Check sheet for the modelled part. Datum: model origin and axes. Units: mm. A direction names the side the tool comes from. Coordinates: 2 decimals unless noted, no trailing zeros. Loops run counter-clockwise (first coordinate to the right, second up) from the corner with the lowest first, then second, coordinate; pieces in that order, holes last. Notation, with made-up numbers: M 7,75 L 30,75 A30 cw 30,100 Z; hole C 80,88 d2. An arc over 180 degrees is marked long. Return JSON: item names as keys, results as strings.
from build123d import *

# Parameters (mm, degrees)
F0_W     = 9.52
F0_H     = 4.8375
F1_DEPTH = 1.5
F2_W     = 1.7
F2_H     = 6.7225
F3_DEPTH = 1.501


with BuildPart() as f1:
    # F0 (on Top) → F1 (new body)
    with BuildSketch(Plane.XY):
        with Locations((0, 8.88625)):
            Rectangle(F0_W, F0_H)
        with BuildLine():
            ThreePointArc((17.96, -4.5625), (13.3975, 0), (17.96, 4.5625))
            Line((17.96, 4.5625), (17.96, 6.4675))
            ThreePointArc((17.96, 6.4675), (11.4925, 0), (17.96, -6.4675))
            Line((17.96, -6.4675), (17.96, -4.5625))
        make_face()
        with BuildLine():
            Line((-17.96, -4.5625), (-17.96, -6.4675))
            ThreePointArc((-17.96, -6.4675), (-13.386787, -4.573213), (-11.4925, 0))
            ThreePointArc((-11.4925, 0), (-13.386787, 4.573213), (-17.96, 6.4675))
            Line((-17.96, 6.4675), (-17.96, 4.5625))
            ThreePointArc((-17.96, 4.5625), (-14.733825, 3.226175), (-13.3975, 0))
            ThreePointArc((-13.3975, 0), (-14.733825, -3.226175), (-17.96, -4.5625))
        make_face()
        with BuildLine():
            ThreePointArc((17.96, 4.5625), (21.186175, 3.226175), (22.5225, 0))
            ThreePointArc((22.5225, 0), (21.186175, -3.226175), (17.96, -4.5625))
            Line((17.96, -4.5625), (17.96, -6.4675))
            ThreePointArc((17.96, -6.4675), (22.533213, -4.573213), (24.4275, 0))
            ThreePointArc((24.4275, 0), (22.533213, 4.573213), (17.96, 6.4675))
            Line((17.96, 6.4675), (17.96, 4.5625))
        make_face()
        with BuildLine():
            ThreePointArc((-17.96, 6.4675), (-24.4275, 0), (-17.96, -6.4675))
            Line((-17.96, -6.4675), (-17.96, -4.5625))
            ThreePointArc((-17.96, -4.5625), (-22.5225, 0), (-17.96, 4.5625))
            Line((-17.96, 4.5625), (-17.96, 6.4675))
        make_face()
        with BuildLine():
            ThreePointArc((17.96, -6.4675), (11.4925, 0), (17.96, 6.4675))
            Line((17.96, 6.4675), (4.76, 6.4675))
            Line((4.76, 6.4675), (-4.76, 6.4675))
            Line((-4.76, 6.4675), (-17.96, 6.4675))
            ThreePointArc((-17.96, 6.4675), (-13.386787, 4.573213), (-11.4925, 0))
            ThreePointArc((-11.4925, 0), (-13.386787, -4.573213), (-17.96, -6.4675))
            Line((-17.96, -6.4675), (17.96, -6.4675))
        make_face()
    extrude(amount=F1_DEPTH)

    # F2 (on face) → F3 (cut, through all)
    with BuildSketch(Plane.XY.offset(1.5)):
        with Locations((0, -3.10625)):
            Rectangle(F2_W, F2_H)
    extrude(amount=-F3_DEPTH, mode=Mode.SUBTRACT)


solid = f1.part
1) Set-up check for faces 1 (the face through (0.85, -3, 1)), 2 (the face through (-24.426, 0.142, 0.74)), 3 (the face through (-11, 6.468, 1)), 4 (the face through (11, 6.468, 1)): record each of +Z, -Z, +X, -X, +Y, -Y from which the full face is reachable in a straight line by a thin tool's end or side.
Answers:
{"face 1": "+Z, -Z, -Y", "face 2": "+Z, -Z, -X", "face 3": "+Z, -Z, -X, +Y", "face 4": "+Z, -Z, +X, +Y"}
2) Section check D-D on x = -9. Record the cut outline in (y, z), then the cut area to 3 significant figures.
Answers:
{"outline": "M -6.47,0 L 6.47,0 L 6.47,1.5 L -6.47,1.5 Z", "area": "19.4 mm²"}
3) Go/stop test with flat-tipped pins: pin 1 Ø10 at (x, y) = (12, 4.5) entering from -Z; pin 2 Ø0.8 at (y, z) = (8, 0.5) entering from +X. Record where each tip stops, or that it passes through.
Answers:
{"pin 1": "z = 0", "pin 2": "x = 4.76"}
4) Section check B-B on y = -3.5. Record the cut outline in (x, z), then the cut area to 3 significant figures.
Answers:
{"outline": "M -23.4,0 L -20.89,0 L -20.89,1.5 L -23.4,1.5 Z; M -15.03,0 L -0.85,0 L -0.85,1.5 L -15.03,1.5 Z; M 0.85,0 L 15.03,0 L 15.03,1.5 L 0.85,1.5 Z; M 20.89,0 L 23.4,0 L 23.4,1.5 L 20.89,1.5 Z", "area": "50.1 mm²"}
5) Section check A-A on z = 0.65. Count the separate pieces of the cut face and the enclosed holes in it, then the cut area to 3 significant figures.
Answers:
{"separate pieces": "1", "enclosed holes": "2", "area": "500 mm²"}
6) Section check C-C on y = 7. Record the cut outline in (x, z).
Answers:
{"outline": "M -4.76,0 L 4.76,0 L 4.76,1.5 L -4.76,1.5 Z"}
7) Scan lines: line 1 along X through (y, z) = (-2, 0.1); line 2 along X through (y, z) = (1, 0.7); line 3 along X through (y, z) = (-1.25, 1.4). Record each from-to range of solid material in increasing order. Write a range as [from, to].
Answers:
{"line 1": "[-24.11, -22.06], [-13.86, -0.85], [0.85, 13.86], [22.06, 24.11]", "line 2": "[-24.35, -22.41], [-13.51, 13.51], [22.41, 24.35]", "line 3": "[-24.31, -22.35], [-13.57, -0.85], [0.85, 13.57], [22.35, 24.31]"}
